Geometry: final body of the model. Coordinates: model frame, mm. A direction names the side the tool comes from. Coordinates: 2 decimals unless noted, no trailing zeros. Write each loop counter-clockwise with the first axis right and the second up, starting at its lowest first coordinate (ties: lowest second). Pieces come first, ordered by that corner, then holes. Notation, with made-up numbers: (68, -18.75) -> (121, -18.75) arc R28 ccw to (121, 7.25) -> close; hole circle Ø6 at (-8, -25.5). An arc over 180 degrees is marked (long way). One line per item, written item: value.
```python
from build123d import *

# Parameters (mm, degrees)
SKETCH1_R           = 8.4935
BOSS_EXTRUDE1_DEPTH = 12
SKETCH2_R           = 2.5
CUT_EXTRUDE1_DEPTH  = 10.5
CUT_EXTRUDE2_DEPTH  = 20
FILLET1_R           = 4.85


with BuildPart() as part:
    # Sketch1 → Boss-Extrude1 (new body)
    with BuildSketch(Plane(origin=(0, 0, 0), x_dir=(1, 0, 0), z_dir=(0, 1, 0))):
        with BuildLine():
            Line((-11.9935, 0), (-11.9935, -1))
            Line((-11.9935, -1), (-17.270132019, -5.684762464))
            Line((-17.270132019, -5.684762464), (-17.270132019, -17.9935))
            Line((-17.270132019, -17.9935), (-16, -17.9935))
            Line((-16, -17.9935), (16, -17.9935))
            Line((16, -17.9935), (17.270132019, -17.9935))
            Line((17.270132019, -17.9935), (17.270132019, -5.684762464))
            Line((17.270132019, -5.684762464), (11.9935, -1))
            Line((11.9935, -1), (11.9935, 0))
            ThreePointArc((11.9935, 0), (0, 11.9935), (-11.9935, 0))
        make_face()
        with Locations(Location((0, 0, 0), (0, 0, 270))):
            Circle(SKETCH1_R, mode=Mode.SUBTRACT)
    extrude(amount=BOSS_EXTRUDE1_DEPTH)

    # Sketch2 → Cut-Extrude1 (cut)
    with BuildSketch(Plane.XY.offset(17.9935)):
        with Locations((-11.811421167, 6)):
            Circle(SKETCH2_R)
        with Locations((11.811421167, 6)):
            Circle(SKETCH2_R)
    extrude(amount=-CUT_EXTRUDE1_DEPTH, mode=Mode.SUBTRACT)

    # Sketch3 → Cut-Extrude2 (cut)
    with BuildSketch(Plane(origin=(0, 12, 0), x_dir=(1, 0, 0), z_dir=(0, 1, 0))):
        with BuildLine():
            Line((-6.25, -17.9935), (-6.25, -8.738437632))
            ThreePointArc((-6.25, -8.738437632), (0.155303572, -10.742377439), (6.5, -8.55410967))
            Line((6.5, -8.55410967), (6.5, -17.9935))
            Line((6.5, -17.9935), (-6.25, -17.9935))
        make_face()
    extrude(amount=-CUT_EXTRUDE2_DEPTH, mode=Mode.SUBTRACT)

    # Fillet1
    fillet1_edges = [part.edges().sort_by_distance(p)[0] for p in [
        (6.5, 6, 8.55410967),
        (-6.25, 6, 8.738437632),
        (-17.270132019, 6, 5.684762464),
        (-11.9935, 6, 1),
        (11.9935, 6, 1),
        (17.270132019, 6, 5.684762464),
    ]]
    fillet(fillet1_edges, radius=FILLET1_R)


solid = part.part
```
(1) Reachability of faces 5 (the flat face through (12, 6, 7.494)), 6 (the flat face through (-6.25, 6, 17)), 7 (the cylindrical face through (0.25, 5.92, -11.99)) from +Z, -Z, +X, -X, +Y, -Y: full face, straight path, thin tool, end or side. Return the list, or none.
Responses:
face 5: +Z
face 6: +Z, +Y, -Y
face 7: -Z, +Y, -Y
(2) Line query: line 1 (X direction, y = 7, z = -2.5); line 2 (X direction, y = 7, z = 0) (1 decimal); line 3 (X direction, y = 7.25, z = 13.25). Output: solid intervals per line, ascending. Write a range as [from, to].
Responses:
line 1: x = [-11.73, -8.12], [8.12, 11.73]
line 2: x = [-12.1, -8.5], [8.5, 12.1]
line 3: x = [-17.27, -13.98], [-9.65, -5.68], [5.94, 9.65], [13.98, 17.27]
(3) Section C-C (x = 15). Return the cut outline in (y, z), then the cut area to 3 significant figures.
Responses:
outline: (0, 3.67) -> (12, 3.67) -> (12, 17.99) -> (0, 17.99) -> close
area: 172 mm2
(4) Section A-A (x = 0). Return the cut outline in (y, z), then the cut area to 3 significant figures.
Responses:
outline: (0, -11.99) -> (12, -11.99) -> (12, -8.49) -> (0, -8.49) -> close; (0, 8.49) -> (12, 8.49) -> (12, 10.74) -> (0, 10.74) -> close
area: 69.0 mm2
(5) Section B-B (z = -7.25). Return the cut outline in (x, y), then the cut area to 3 significant figures.
Responses:
outline: (-9.55, 0) -> (-4.42, 0) -> (-4.42, 12) -> (-9.55, 12) -> close; (4.42, 0) -> (9.55, 0) -> (9.55, 12) -> (4.42, 12) -> close
area: 123 mm2
(6) First-contact query: pin 1 (4.5 mm diameter, centred on x = -11.81, y = 6, fed in from -Z); pin 2 (1.5 mm diameter, centred on y = 8, z = -4.5, fed in from +X); pin 3 (3 mm diameter, centred on x = -8, y = 2, fed in from -Z). Flat tips, straight axial feed; report the tip coordinate or a pass-through.
Responses:
pin 1: stops at z = -7.24
pin 2: stops at x = 11.39
pin 3: stops at z = -10.08
(7) Pull-direction query (X, two-part tool) for faces 1 (the flat face through (12, 3, 17.994)), 2 (the flat face through (6.5, 6, 17)), 3 (the cylindrical face through (16.83, 6.08, 5.85)), 4 (the cylindrical face through (-9.427, 6.751, 12.817)); classes: released by +X, released by -X, zero draft, split by the parting line, or undercut.
Responses:
face 1: zero draft
face 2: undercut
face 3: released by +X
face 4: undercut
